For this review, use the dimensioned drawing (mm, ordinates from the lowest corner) and the shaded views. A direction names the side the tool comes from. Round coordinates to 2 decimals unless told otherwise and drop trailing zeros. Write each loop counter-clockwise with the first axis right and the second up, starting at its lowest first coordinate (ties: lowest second). Pieces come first, ordered by that corner, then holes. Notation, with made-up numbers: (40, -21.75) - (63, -21.75) arc R32 ccw to (63, 10.25) - close; hole circle Ø10 at (14, 50.25). An arc over 180 degrees is marked (long way). Write each question's results on one line, items separated by ' | '.
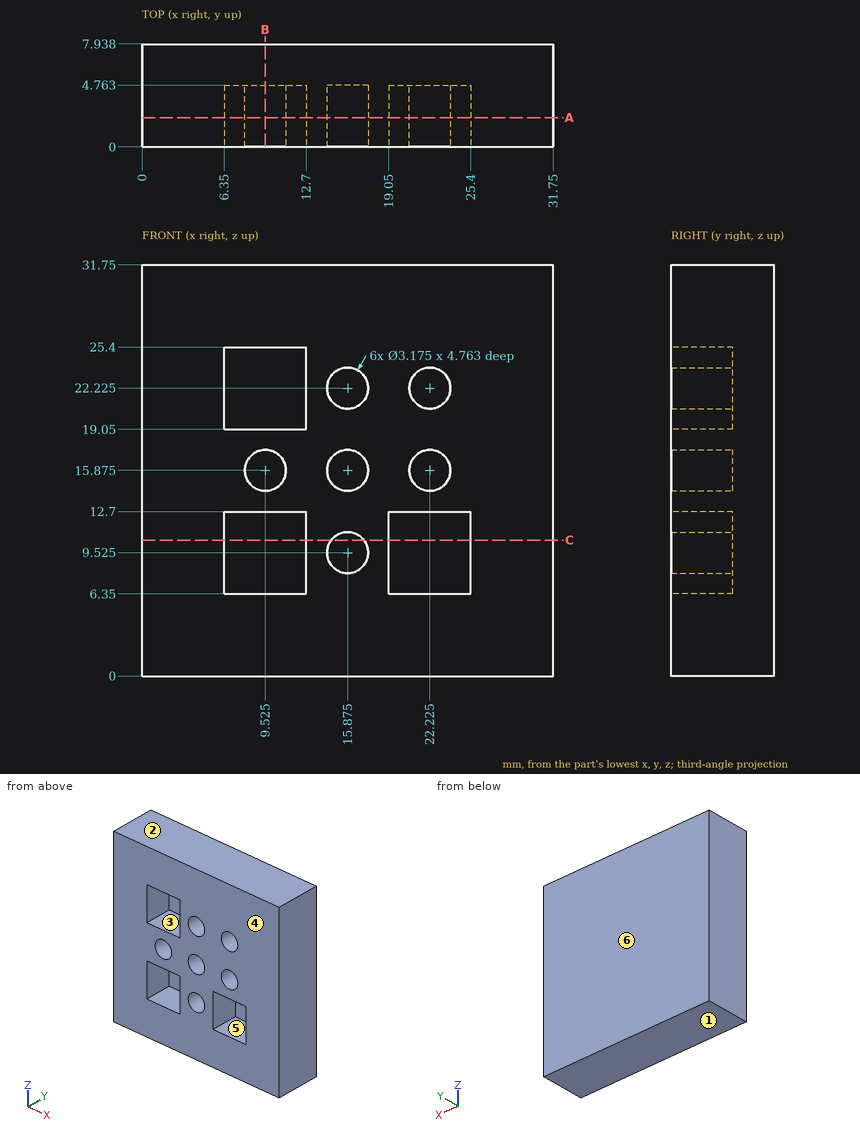
Q1. We need section A-A (y = 2.25). State how many separate pieces and enclosed holes the cut face has.
Evaluation:
separate pieces: 1 | enclosed holes: 9
Q2. We need section C-C (z = 10.5). State the section outline as (x, y) points.
Evaluation:
outline: (0, 0) - (6.35, 0) - (6.35, 4.76) - (12.7, 4.76) - (12.7, 0) - (14.62, 0) - (14.62, 4.76) - (17.13, 4.76) - (17.13, 0) - (19.05, 0) - (19.05, 4.76) - (25.4, 4.76) - (25.4, 0) - (31.75, 0) - (31.75, 7.94) - (0, 7.94) - close
Q3. For probe 1 along X at (y, z) = (3.5, 16); probe 2 along Z at (x, y) = (12, 3.75); probe 3 along Z at (x, y) = (9, 0.5), list the stretches that pass through material, from the lowest coordinate up.
Evaluation:
probe 1: x = 0 to 7.94, 11.11 to 14.29, 17.46 to 20.64, 23.81 to 31.75 | probe 2: z = 0 to 6.35, 12.7 to 19.05, 25.4 to 31.75 | probe 3: z = 0 to 6.35, 12.7 to 14.38, 17.37 to 19.05, 25.4 to 31.75
Q4. We need section B-B (x = 9.5). State the section outline as (y, z) points.
Evaluation:
outline: (0, 0) - (7.94, 0) - (7.94, 31.75) - (0, 31.75) - (0, 25.4) - (4.76, 25.4) - (4.76, 19.05) - (0, 19.05) - (0, 17.46) - (4.76, 17.46) - (4.76, 14.29) - (0, 14.29) - (0, 12.7) - (4.76, 12.7) - (4.76, 6.35) - (0, 6.35) - close
Q5. Insertion check: P1, Ø1.9, axis at x = 9.525, z = 15.875, coming from the -Y side. The pin has a flat end and moves straight along its axis. Give the tip position at first contact, or say it passes through.
Evaluation:
P1: stops at y = 4.76
Q6. Tool access review of the marked faces 5 and 6: name each direction out of +Z, -Z, +X, -X, +Y, -Y from which nothing blocks a thin tool from reaching the whole face with its end or side.
Evaluation:
face 5: -Y | face 6: +Z, -Z, +X, -X, +Y
Q7. The part is to be moulded in two halves that separate along Z. For the marked faces 1, 2, 3 and 4, say which applies: released by +Z, released by -Z, zero draft, split by the parting line, or undercut.
Evaluation:
face 1: released by -Z | face 2: released by +Z | face 3: undercut | face 4: zero draft
